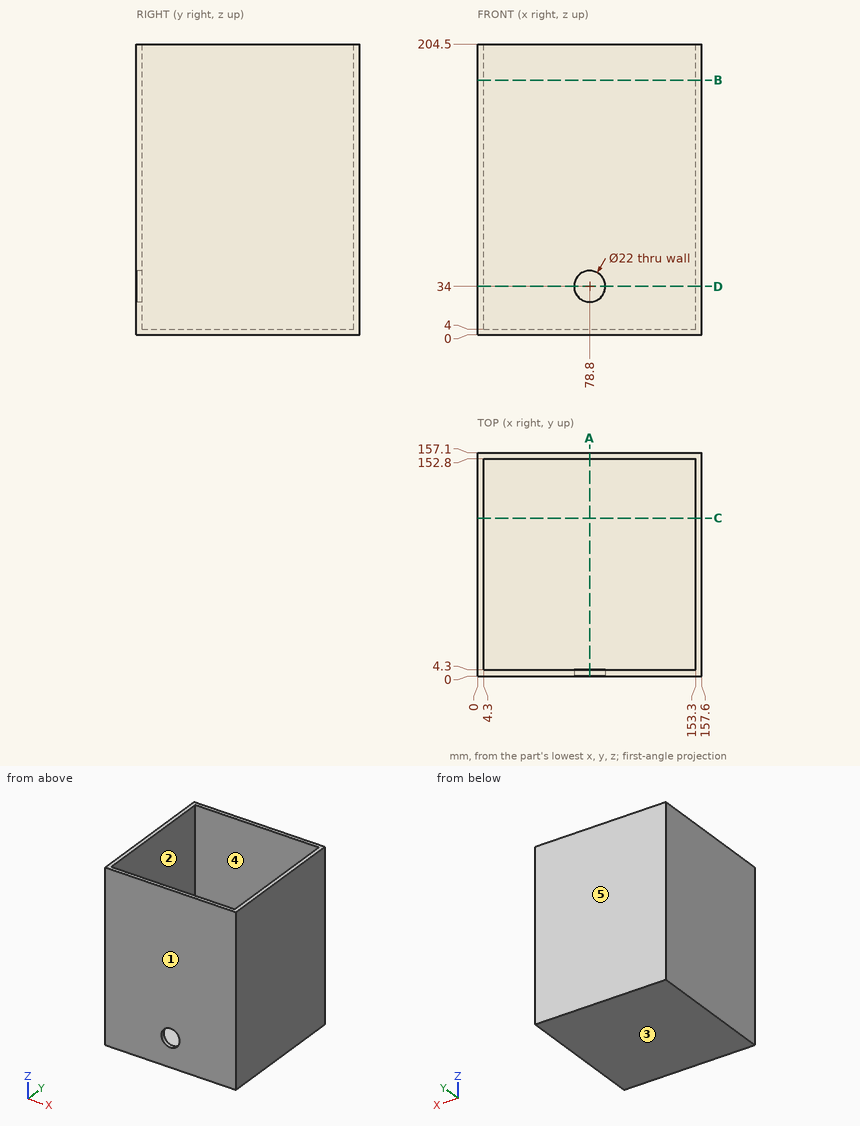
Source: three-view drawing plus pictorial views. Frame: mm from the lowest corner of the part. A direction names the side the tool comes from. Round coordinates to 2 decimals unless told otherwise and drop trailing zeros. Loops run counter-clockwise (first coordinate to the right, second up) from the corner with the lowest first, then second, coordinate; pieces in that order, holes last.
Q1. Section D-D on z = 34. Return loops of the section in (x, y).
Q2. Material intervals for L1, parallel to X at y = 111, z = 184.5; L2, parallel to Y at x = 139.5, z = 22.5; L3, parallel to X at y = 2.1, z = 34, sorted ascending.
Q3. Pin query (flat end, axial travel): P1, Ø12, axis at x = 121.5, y = 27, coming from the +Z side. Return the tip coordinate at first contact, or that it passes through.
Q4. Access query for the marked faces 1 and 2. Directions: +Z, -Z, +X, -X, +Y, -Y. A direction counts if a zero-diameter tool reaches every point of the face in a straight line with its end or side. Return the directions, or none.
Q5. Section C-C on y = 111. Return loops of the section in (x, z).
Q6. Section B-B on z = 179. Return loops of the section in (x, y), plus the area to 3 significant figures.
Q7. Section A-A on x = 78.8. Return loops of the section in (y, z), plus the area to 3 significant figures.
Q8. Pull-direction query (Y, two-part tool) for the marked faces 3, 4 and 5; classes: released by +Y, released by -Y, zero draft, split by the parting line, or undercut.
Evaluation:
1. outline: (0, 0) - (67.8, 0) - (67.8, 4.3) - (4.3, 4.3) - (4.3, 152.8) - (153.3, 152.8) - (153.3, 4.3) - (89.8, 4.3) - (89.8, 0) - (157.6, 0) - (157.6, 157.1) - (0, 157.1) - close
2. L1: x = 0 to 4.3, 153.3 to 157.6
2. L2: y = 0 to 4.3, 152.8 to 157.1
2. L3: x = 0 to 67.8, 89.8 to 157.6
3. P1: stops at z = 4
4. face 1: +Z, -Z, +X, -X, -Y
4. face 2: +Z
5. outline: (0, 0) - (157.6, 0) - (157.6, 204.5) - (153.3, 204.5) - (153.3, 4) - (4.3, 4) - (4.3, 204.5) - (0, 204.5) - close
6. outline: (0, 0) - (157.6, 0) - (157.6, 157.1) - (0, 157.1) - close; hole (4.3, 4.3) - (153.3, 4.3) - (153.3, 152.8) - (4.3, 152.8) - close
6. area: 2,630 mm2
7. outline: (0, 0) - (157.1, 0) - (157.1, 204.5) - (152.8, 204.5) - (152.8, 4) - (4.3, 4) - (4.3, 23) - (0, 23) - close; (0, 45) - (4.3, 45) - (4.3, 204.5) - (0, 204.5) - close
7. area: 2,260 mm2
8. face 3: zero draft
8. face 4: undercut
8. face 5: released by +Y
